```python
from build123d import *

# Parameters (mm, degrees)
SZKIC2_R                    = 30.5
DODANIE_WYCI_GNI_CIE2_DEPTH = 6
OTW_R_9_0_9_1_D             = 9
SZKIC8_R                    = 6.5
WYTNIJ_WYCI_GNI_CIE2_DEPTH  = 6


with BuildPart() as part:
    # Szkic2 → Dodanie-wyciągnięcie2 (new body)
    with BuildSketch(Plane(origin=(0, 0, 0), x_dir=(1, 0, 0), z_dir=(0, 1, 0))):
        with Locations(Location((0, 0, 0), (0, 0, 270))):
            Circle(SZKIC2_R)
    extrude(amount=DODANIE_WYCI_GNI_CIE2_DEPTH)

    # Otwór Ø9.0 (9)1 (through all)
    with Locations(Plane(origin=(0, 6, 0), x_dir=(1, 0, 0), z_dir=(0, 1, 0))):
        with Locations((0, 0)):
            Hole(OTW_R_9_0_9_1_D / 2)

    # Szkic8 → Wytnij-wyciągnięcie2 (cut)
    with BuildSketch(Plane(origin=(0, 6, 0), x_dir=(1, 0, 0), z_dir=(0, 1, 0))):
        with Locations(Location((-12.751231108, -11.985662487, 0), (0, 0, 270))):
            Circle(SZKIC8_R)
        with Locations(Location((-16.755503748, 5.050058825, 0), (0, 0, 270))):
            Circle(SZKIC8_R)
        with Locations(Location((-4.004272641, 17.035721312, 0), (0, 0, 270))):
            Circle(SZKIC8_R)
        with Locations(Location((12.751231108, 11.985662487, 0), (0, 0, 270))):
            Circle(SZKIC8_R)
        with Locations(Location((16.755503748, -5.050058825, 0), (0, 0, 270))):
            Circle(SZKIC8_R)
        with Locations(Location((4.004272641, -17.035721312, 0), (0, 0, 270))):
            Circle(SZKIC8_R)
    extrude(amount=-WYTNIJ_WYCI_GNI_CIE2_DEPTH, mode=Mode.SUBTRACT)


solid = part.part
```
Geometry: final body of the model. Coordinates: model frame, mm. Give positions to 0.01 mm unless a question says otherwise; leave off trailing zeros. Loops run counter-clockwise (first coordinate to the right, second up) from the corner with the lowest first, then second, coordinate; pieces in that order, holes last. Notation, with made-up numbers: (79.25, 42.5) -> (103.25, 42.5) arc R16 ccw to (103.25, 63.5) -> close; hole circle Ø5 at (10, 12.5). An arc over 180 degrees is marked (long way). Use CSV: the item, a comma, the result in double quotes.
(1) First-contact query: P1, Ø2, axis at y = 5, z = 16, coming from the -X side; P2, Ø11.5, axis at x = 0, z = 0, coming from the +Y side; P3, Ø3, axis at y = 1.5, z = 23.5, coming from the -X side. Flat tips, straight axial feed; report the tip coordinate or a pass-through.
From the geometry:
P1,"x = -26.56"
P2,"y = 6"
P3,"x = -21.12"
(2) Cut plane C-C (y = 1.15). Output: boundary loops of the cut face in (x, z), plus the area to 3 significant figures.
From the geometry:
outline,"circle Ø61 at (0, 0); hole circle Ø13 at (-16.76, -5.05); hole circle Ø13 at (-12.75, 11.99); hole circle Ø13 at (-4, -17.04); hole circle Ø9 at (0, 0); hole circle Ø13 at (4, 17.04); hole circle Ø13 at (12.75, -11.99); hole circle Ø13 at (16.76, 5.05)"
area,"2,060 mm^2"
(3) Pull-direction query (Z, two-part tool) for faces 1 (the face through (-2.052, 3.042, -10.836)), 2 (the face through (-23.1, 3.04, -6.46)), 3 (the face through (0, 0, 6)), 4 (the face through (-29.775, 2.958, -6.612)); classes: released by +Z, released by -Z, zero draft, split by the parting line, or undercut.
From the geometry:
face 1,"undercut"
face 2,"undercut"
face 3,"zero draft"
face 4,"split by the parting line"
(4) Cut plane B-B (z = 14.5). Output: boundary loops of the cut face in (x, y), plus the area to 3 significant figures.
From the geometry:
outline,"(-26.83, 0) -> (-18.75, 0) -> (-18.75, 6) -> (-26.83, 6) -> close; (-6.76, 0) -> (-1.98, 0) -> (-1.98, 6) -> (-6.76, 6) -> close; (9.99, 0) -> (26.83, 0) -> (26.83, 6) -> (9.99, 6) -> close"
area,"178 mm^2"
(5) Ray query, line 1 along Z through (x, y) = (7, 5.7); line 2 along Z through (x, y) = (-16, 2.35); line 3 along X through (y, z) = (3.35, 15.5). Return the intervals inside material, ascending. Write a range as [from, to].
From the geometry:
line 1,"[-29.69, -15.01], [-8.96, 11.27], [22.8, 29.69]"
line 2,"[-25.97, -11.51], [1.41, 6.36], [17.62, 25.97]"
line 3,"[-26.27, -18.22], [-7.28, -2.31], [10.32, 26.27]"
(6) Cut plane A-A (x = 1.5). Output: boundary loops of the cut face in (y, z).
From the geometry:
outline,"(0, -30.46) -> (6, -30.46) -> (6, -20.49) -> (0, -20.49) -> close; (0, -13.58) -> (6, -13.58) -> (6, -4.24) -> (0, -4.24) -> close; (0, 4.24) -> (6, 4.24) -> (6, 11.04) -> (0, 11.04) -> close; (0, 23.03) -> (6, 23.03) -> (6, 30.46) -> (0, 30.46) -> close"
(7) Cut plane D-D (x = -8). Output: boundary loops of the cut face in (y, z).
From the geometry:
outline,"(0, -29.43) -> (6, -29.43) -> (6, -22.16) -> (0, -22.16) -> close; (0, -11.91) -> (6, -11.91) -> (6, 7.55) -> (0, 7.55) -> close; (0, 16.42) -> (6, 16.42) -> (6, 29.43) -> (0, 29.43) -> close"
